from build123d import *

# Parameters (mm, degrees)
CUT_EXTRUDE1_DEPTH  = 5
CUT_EXTRUDE11_DEPTH = 5


with BuildPart() as part:
    # Sketch1 → Revolve1 (revolve)
    with BuildSketch(Plane(origin=(0, 0, 0), x_dir=(1, 0, 0), z_dir=(0, 1, 0)), mode=Mode.PRIVATE) as revolve1_sk:
        Polygon((0, 0), (0, -265), (17, -265), (17, -245), (20, -245), (20, -95), (16, -95), (16, -45), (15, -45), (15, 0), align=None)
    revolve(revolve1_sk.sketch.rotate(Axis((0, 0, 0), (0, 0, 1)), 180), axis=Axis((0, 0, 0), (0, 0, 1)))

    # Sketch3 → Cut-Extrude1 (cut)
    with BuildSketch(Plane(origin=(2.233419524, 16, 45), x_dir=(0, 0, -1), z_dir=(0, -1, 0))):
        with BuildLine():
            Line((-10, 2.766580476), (-40, 2.766580476))
            ThreePointArc((-40, 2.766580476), (-45, -2.233419524), (-40, -7.233419524))
            Line((-40, -7.233419524), (-10, -7.233419524))
            ThreePointArc((-10, -7.233419524), (-5, -2.233419524), (-10, 2.766580476))
        make_face()
    extrude(amount=CUT_EXTRUDE1_DEPTH, mode=Mode.SUBTRACT)

    # Sketch31 → Cut-Extrude11 (cut)
    with BuildSketch(Plane(origin=(1.137793825, 20, 245), x_dir=(0, 0, 1), z_dir=(0, -1, 0))):
        with BuildLine():
            Line((-30, 7.137793825), (-90, 7.137793825))
            ThreePointArc((-90, 7.137793825), (-96, 1.137793825), (-90, -4.862206175))
            Line((-90, -4.862206175), (-30, -4.862206175))
            ThreePointArc((-30, -4.862206175), (-24, 1.137793825), (-30, 7.137793825))
        make_face()
    extrude(amount=CUT_EXTRUDE11_DEPTH, mode=Mode.SUBTRACT)


solid = part.part
Build history of the part. All positions in model axes, mm. A direction names the side the tool comes from. Coordinates: 2 decimals unless noted, no trailing zeros. Order: outer loops, then holes, each group sorted by start corner. A loop starts at its lowest first (then second) coordinate and runs counter-clockwise, first axis right, second up. Notation, with made-up numbers: (6, -0.75) -> (46, -0.75) arc R25 cw to (46, 18.25) -> close; hole circle Ø7 at (23.5, 1). An arc over 180 degrees is marked (long way). One line per item, written item: value.
(1) Slice it at A-A, the plane x = -9. List the corners of the cut face in (y, z), plus the area to 3 significant figures.
Checked values:
outline: (-17.86, 95) -> (-13.23, 95) -> (-13.23, 45) -> (-12, 45) -> (-12, 0) -> (12, 0) -> (12, 45) -> (13.23, 45) -> (13.23, 95) -> (17.86, 95) -> (17.86, 245) -> (14.42, 245) -> (14.42, 265) -> (-14.42, 265) -> (-14.42, 245) -> (-17.86, 245) -> close
area: 8,340 mm2
(2) Tool access for faces 1 (the cylindrical face through (0, 14, 90)), 2 (the flat face through (0, 0, 0)), 3 (the cylindrical face through (2.213, -16.855, 254.86)), 4 (the cylindrical face through (-8.6, -13.49, 69.65)): list every direction of +Z, -Z, +X, -X, +Y, -Y with a clear straight run to the whole face (end or side of a thin tool).
Checked values:
face 1: +Y
face 2: -Z, +X, -X, +Y, -Y
face 3: +Z
face 4: -Z
(3) Slice it at B-B, the plane y = -5.5. List the corners of the cut face in (x, z).
Checked values:
outline: (-19.23, 95) -> (-15.02, 95) -> (-15.02, 45) -> (-13.96, 45) -> (-13.96, 0) -> (13.96, 0) -> (13.96, 45) -> (15.02, 45) -> (15.02, 95) -> (19.23, 95) -> (19.23, 245) -> (16.09, 245) -> (16.09, 265) -> (-16.09, 265) -> (-16.09, 245) -> (-19.23, 245) -> close
(4) Drop flat-ended pins along their axis: pin 1 Ø11 at (x, z) = (-2, 65.5) entering from +Y; pin 2 Ø2 at (x, z) = (-13, 230.5) entering from -Y; pin 3 Ø2 at (y, z) = (13, 71) entering from -X. Give the stop position or say it passes through.
Checked values:
pin 1: y = 15.2
pin 2: y = -16
pin 3: x = -10.58
(5) Slice it at C-C, the plane z = 76. List the corners of the cut face in (x, y).
Checked values:
outline: (-5, 11) -> (-5, 15.2) arc R16 ccw (long way) to (5, 15.2) -> (5, 11) -> close
(6) Mould opens along Z. For faces 5 (the flat face through (-9, 15, 245)), 6 (the flat face through (8.98, -13.43, 95)), 7 (the cylindrical face through (0, 18, 149)) say: pulls with the +Z half, pulls with the -Z half, needs draft (parallel to the pull), parting line crosses it, or undercut.
Checked values:
face 5: pulls with the +Z half
face 6: pulls with the -Z half
face 7: undercut
(7) Probe line 1 (X direction, y = 12, z = 198.5); line 2 (Y direction, x = -1, z = 129); line 3 (Z direction, x = 6, y = -14.5). List the from-to ranges inside material, lowest first. Write a range as [from, to].
Checked values:
line 1: [-16, 16]
line 2: [-19.97, 19.97]
line 3: [45, 265]
(8) Slice it at D-D, the plane z = 210. List the corners of the cut face in (x, y).
Checked values:
outline: (-6, 15) -> (-6, 19.08) arc R20 ccw (long way) to (6, 19.08) -> (6, 15) -> close
